```python
from build123d import *

# Parameters (mm, degrees)
BOSS_EXTRUDE1_DEPTH     = 17.5
BOSS_EXTRUDE2_DEPTH     = 6.5
SKETCH4_W               = 24.52025143
SKETCH4_H               = 35
CUT_EXTRUDE1_DEPTH      = 3.5
SKETCH5_W               = 23.62971737
SKETCH5_H               = 2
CUT_EXTRUDE2_DEPTH      = 4.5
FILLET1_R               = 5
SKETCH7_W               = 9
SKETCH7_H               = 4
SKETCH7_W_2             = 8.890538969
SKETCH7_H_2             = 3.998522236
BOSS_EXTRUDE3_DEPTH     = 6.5
FILLET2_R               = 1
CUT_EXTRUDE4_REACH      = 69.415
SKETCH8_W               = 18
SKETCH8_H               = 16
FILLET3_R               = 0.5
CUT_EXTRUDE5_REACH      = 69.415
SKETCH9_W               = 18
SKETCH9_H               = 16
FILLET4_R               = 0.5
SKETCH10_W              = 28.52025143
SKETCH10_H              = 6.445257338
CUT_EXTRUDE6_DEPTH      = 3
CUT_EXTRUDE7_DEPTH      = 10
CUT_EXTRUDE7_DEPTH_BACK = 68.853985243


with BuildPart() as part:
    # Sketch1 → Boss-Extrude1 (new body)
    with BuildSketch(Plane.XY):
        Polygon((0.056027157, 6.000000005), (14.056027157, 6.000000005), (14.056027157, 41.000000005), (38.576278587, 41.000000005), (38.576278587, 6.000000005), (52.466817556, 6.000000005), (52.576278587, 9.99850201), (43.576278587, 9.998522241), (43.576278587, 39.558678923), (43.576278587, 45.550000005), (41.466812647, 45.550000005), (38.316152872, 45.550000005), (14.316152872, 45.550000005), (9.056027157, 45.550000005), (9.056027157, 39.558678923), (9.056027157, 10.000000005), (0.056027157, 10.000000005), align=None)
    extrude(amount=BOSS_EXTRUDE1_DEPTH)

    # Sketch2 → Boss-Extrude2 (add)
    with BuildSketch(Plane.XY.offset(17.5)):
        Polygon((9.056027157, 10.000000005), (9.056027157, 45.550000005), (43.576278587, 45.550000005), (43.576278587, 6.000000005), (9.056027157, 6.000000005), align=None)
    extrude(amount=BOSS_EXTRUDE2_DEPTH)

    # Sketch4 → Cut-Extrude1 (cut)
    with BuildSketch(Plane(origin=(0, 0, 17.5), x_dir=(-1, 0, 0), z_dir=(0, 0, -1))):
        with Locations((-26.316152872, 23.500000005)):
            Rectangle(SKETCH4_W, SKETCH4_H)
    extrude(amount=-CUT_EXTRUDE1_DEPTH, mode=Mode.SUBTRACT)

    # Sketch5 → Cut-Extrude2 (cut)
    with BuildSketch(Plane(origin=(0, 0, 21), x_dir=(-1, 0, 0), z_dir=(0, 0, -1))):
        with Locations((-26.761419902, 42.000000005)):
            Rectangle(SKETCH5_W, SKETCH5_H)
    extrude(amount=CUT_EXTRUDE2_DEPTH, mode=Mode.SUBTRACT)

    # Fillet1
    fillet1_edges = [part.edges().sort_by_distance(p)[0] for p in [
        (9.056027157, 45.550000005, 12),
        (43.576278587, 45.550000005, 12),
    ]]
    fillet(fillet1_edges, radius=FILLET1_R)

    # Sketch7 → Boss-Extrude3 (add, through all)
    with BuildSketch(Plane.XY.offset(17.5)):
        with Locations((4.556027157, 8.000000005)):
            Rectangle(SKETCH7_W, SKETCH7_H)
        with Locations((48.021548072, 7.999261123)):
            Rectangle(SKETCH7_W_2, SKETCH7_H_2)
    extrude(amount=BOSS_EXTRUDE3_DEPTH)

    # Fillet2
    fillet2_edges = [part.edges().sort_by_distance(p)[0] for p in [
        (38.576278587, 23.500000005, 0),
        (14.056027157, 23.500000005, 0),
    ]]
    fillet(fillet2_edges, radius=FILLET2_R)

    # Sketch8 → Cut-Extrude4 (cut, up to next)
    with BuildSketch(Plane.ZY.offset(-9.056027157), mode=Mode.PRIVATE) as cut_extrude4_sk1:
        with Locations((12, 30.550000005)):
            Rectangle(SKETCH8_W, SKETCH8_H)
    cut_extrude4_tool1 = extrude(cut_extrude4_sk1.sketch, amount=-CUT_EXTRUDE4_REACH, mode=Mode.PRIVATE) & part.part
    add(cut_extrude4_tool1.solids().sort_by_distance((9.056027, 30.55, 12))[0], mode=Mode.SUBTRACT)

    # Fillet3
    fillet3_edges = [part.edges().sort_by_distance(p)[0] for p in [
        (14.056027157, 30.550000005, 3),
        (14.056027157, 22.550000005, 12),
        (11.556027157, 22.550000005, 21),
        (9.056027157, 30.550000005, 3),
        (9.056027157, 22.550000005, 12),
        (9.056027157, 30.550000005, 21),
        (9.056027157, 38.550000005, 12),
        (14.056027157, 14.275000005, 21),
    ]]
    fillet(fillet3_edges, radius=FILLET3_R)

    # Sketch9 → Cut-Extrude5 (cut, up to next)
    with BuildSketch(Plane(origin=(43.576278587, 0, 0), x_dir=(0, 0, -1), z_dir=(1, 0, 0)), mode=Mode.PRIVATE) as cut_extrude5_sk1:
        with Locations((-12, 30.550000005)):
            Rectangle(SKETCH9_W, SKETCH9_H)
    cut_extrude5_tool1 = extrude(cut_extrude5_sk1.sketch, amount=-CUT_EXTRUDE5_REACH, mode=Mode.PRIVATE) & part.part
    add(cut_extrude5_tool1.solids().sort_by_distance((43.576279, 30.55, 12))[0], mode=Mode.SUBTRACT)

    # Fillet4
    fillet4_edges = [part.edges().sort_by_distance(p)[0] for p in [
        (38.576278587, 14.275000005, 21),
        (38.576278587, 38.550000005, 12),
        (38.576278587, 30.550000005, 3),
        (38.576278587, 22.550000005, 12),
        (41.076278587, 22.550000005, 21),
        (43.576278587, 30.550000005, 21),
        (43.576278587, 22.550000005, 12),
        (43.576278587, 30.550000005, 3),
        (43.576278587, 38.550000005, 12),
    ]]
    fillet(fillet4_edges, radius=FILLET4_R)

    # Sketch10 → Cut-Extrude6 (cut)
    with BuildSketch(Plane.XY.offset(24)):
        with Locations((26.316152872, 15.429934293)):
            Rectangle(SKETCH10_W, SKETCH10_H)
    extrude(amount=-CUT_EXTRUDE6_DEPTH, mode=Mode.SUBTRACT)

    # Sketch6 → Cut-Extrude7 (cut, two sides: drawn at the far end of the back side and taken through both)
    with BuildSketch(Plane(origin=(2.2475e-05, 9.998620193, 0), x_dir=(0.9999999999974737, -2.2478262975890884e-06, 0), z_dir=(2.2478262975890884e-06, 0.9999999999974737, 0)).offset(-CUT_EXTRUDE7_DEPTH_BACK)):
        Polygon((4.056004679, -22), (6.556004679, -20.556624327), (6.556004679, -17.669872981), (4.056004679, -16.226497308), (1.556004679, -17.669872981), (1.556004679, -20.556624327), align=None)
        Polygon((1.556004679, -3.450509855), (4.056004679, -2.007134182), (6.556004679, -3.450509855), (6.556004679, -6.337261201), (4.056004679, -7.780636874), (1.556004679, -6.337261201), align=None)
        Polygon((46.576256112, -3.429667879), (49.076256112, -1.986292206), (51.576256112, -3.429667879), (51.576256112, -6.316419225), (49.076256112, -7.759794898), (46.576256112, -6.316419225), align=None)
        Polygon((49.076256112, -22), (51.576256112, -20.556624327), (51.576256112, -17.669872981), (49.076256112, -16.226497308), (46.576256112, -17.669872981), (46.576256112, -20.556624327), align=None)
    extrude(amount=CUT_EXTRUDE7_DEPTH + CUT_EXTRUDE7_DEPTH_BACK, mode=Mode.SUBTRACT)


solid = part.part
```
Here's how the part is built. I have some questions about the finished solid (model axes, mm). A direction names the side the tool comes from. Give positions to 0.01 mm unless a question says otherwise; leave off trailing zeros. Order: outer loops, then holes, each group sorted by start corner. A loop starts at its lowest first (then second) coordinate and runs counter-clockwise, first axis right, second up. Notation, with made-up numbers: (-17, 54) - (23, 54) arc R22 ccw to (23, 74) - close; hole circle Ø4 at (-37.5, 78.25). An arc over 180 degrees is marked (long way). Answer as a JSON object with one key per item and string values. Group by question number.
Item 1: If we section it at A-A on x = 27: Please give me the cut outline in (y, z), and give its area (3 significant figures).
Item 2: If we mould it in two halves opening along Z, with no side actions, what happens to faces 1 (the flat face through (26, 18.653, 23)), 2 (the flat face through (41, 38.55, 12)), 3 (the flat face through (12, 22.55, 12)), 4 (the flat face through (12.6, 25.9, 0))? For each: pulls with the +Z half, pulls with the -Z half, needs draft (parallel to the pull), parting line crosses it, or undercut.
Item 3: If we section it at C-C on z = 15.25: Give the number of separate pieces and of enclosed holes in the cut face, and give its area (3 significant figures).
Item 4: For P1, Ø10.5, axis at x = 25, z = 11.5, coming from the -Y side; P2, Ø3, axis at x = 6.5, y = 28, coming from the +Z side; P3, Ø1.2, axis at x = 10.5, z = 8.5, coming from the +Y side; P4, Ø10, axis at y = 22.5, z = 8, coming from the -X side, each with a flat end and sliding along its axis, tell me the tip position at first contact or that it passes through.
Item 5: Please list where these lines run through material, in increasing order: probe 1 along X at (y, z) = (14, 18.5); probe 2 along Y at (x, z) = (37, 21.5); probe 3 along Z at (x, y) = (40, 18).
Item 6: If we section it at B-B on y = 18: Please give me the cut outline in (x, z).
Item 7: Which directions (+Z, -Z, +X, -X, +Y, -Y) give clear straight access to the entire face, cutting with the end or side of a thin tool? Please do faces 5 (the flat face through (40.576, 15, 23)), 6 (the flat face through (14.947, 42, 19)), 7 (the flat face through (0.056, 8, 12)).
Item 8: If we section it at D-D on y = 24: Please give me the cut outline in (x, z), and give its area (3 significant figures).
Result set:
{
 "1": {"outline": "(6, 21) - (12.21, 21) - (12.21, 24) - (6, 24) - close; (18.65, 21) - (43, 21) - (43, 16.5) - (41, 16.5) - (41, 0) - (45.55, 0) - (45.55, 24) - (18.65, 24) - close", "area": "186 mm²"},
 "2": {"face 1": "needs draft", "face 2": "undercut", "face 3": "undercut", "face 4": "pulls with the -Z half"},
 "3": {"separate pieces": "3", "enclosed holes": "0", "area": "408 mm²"},
 "4": {"P1": "y = 41", "P2": "through", "P3": "y = 44.58", "P4": "x = 9.06"},
 "5": {"probe 1": "9.06 to 14.06, 38.58 to 43.58", "probe 2": "6 to 12.21, 18.65 to 45.55", "probe 3": "0 to 21"},
 "6": {"outline": "(9.06, 0) - (13.06, 0) arc R1 ccw to (14.06, 1) - (14.06, 20.5) arc R0.5 cw to (14.56, 21) - (12.06, 21) - (12.06, 24) - (9.06, 24) - close; (38.08, 21) arc R0.5 cw to (38.58, 20.5) - (38.58, 1) arc R1 ccw to (39.58, 0) - (43.58, 0) - (43.58, 24) - (40.58, 24) - (40.58, 21) - close"},
 "7": {"face 5": "+Z", "face 6": "-Y", "face 7": "+Z, -Z, -X, +Y, -Y"},
 "8": {"outline": "(9.06, 0) - (13.06, 0) arc R1 ccw to (14.06, 1) - (14.06, 2.5) arc R0.5 ccw to (13.56, 3) - (9.56, 3) arc R0.5 ccw to (9.06, 2.5) - close; (9.06, 21.5) arc R0.5 ccw to (9.56, 21) - (43.08, 21) arc R0.5 ccw to (43.58, 21.5) - (43.58, 24) - (9.06, 24) - close; (38.58, 1) arc R1 ccw to (39.58, 0) - (43.58, 0) - (43.58, 2.5) arc R0.5 ccw to (43.08, 3) - (39.08, 3) arc R0.5 ccw to (38.58, 2.5) - close", "area": "133 mm²"}
}
